from build123d import *

# Parameters (mm, degrees)
F0_R     = 49.4073615008
F1_DEPTH = 21.59
F3_D     = 11.5062
F6_D     = 11.5062


with BuildPart() as f1:
    # F0 (on Front) → F1 (new body)
    with BuildSketch(Plane.XZ):
        Circle(F0_R)
    extrude(amount=F1_DEPTH)

    # F3 (through all)
    with Locations(Plane.XZ.offset(21.59)):
        with Locations((-17.7465770394, 17.1450003982)):
            Hole(F3_D / 2)

    # F6 (through all)
    with Locations(Plane.XZ.offset(21.59)):
        with Locations((15.9418433905, 17.1450003982)):
            Hole(F6_D / 2)


solid = f1.part
Input: part model. Units: mm. Frame: model coordinates. Round coordinates to 2 decimals unless told otherwise and drop trailing zeros. Write each loop counter-clockwise with the first axis right and the second up, starting at its lowest first coordinate (ties: lowest second). Pieces come first, ordered by that corner, then holes.
1) Cut plane A-A (z = 13). Return the cut outline in (x, y), then the cut area to 3 significant figures.
2) Draft query along X for faces 1 (the cylindrical face through (47.126, -10.644, 14.841)), 2 (the cylindrical face through (10.63, -10.64, 14.94)), 3 (the flat face through (-1, -21.59, 1)). Return one class per face: pulls with the +X half, pulls with the -X half, needs draft (parallel to the pull), parting line crosses it, or undercut.
3) Cut plane D-D (z = -14.5). Return the cut outline in (x, y), then the cut area to 3 significant figures.
4) Contact query for flat-ended pins moving along their axis: P1, Ø10.5, axis at x = -17.75, z = 17.15, coming from the +Y side; P2, Ø1, axis at y = -6.5, z = -36.5, coming from the -X side; P3, Ø10, axis at x = 31.5, y = -14.5, coming from the +Z side; P4, Ø12, axis at x = -22.5, y = -17.5, coming from the -Z side. Output: stop coordinate, or through.
5) Cut plane C-C (x = 24.5). Return the cut outline in (y, z).
6) Ray query, L1, parallel to X at y = -13.5, z = 19; L2, parallel to X at y = -18, z = 22; L3, parallel to Z at x = -35, y = -3.75. Return the intervals inside material, ascending.
7) Cut plane B-B (y = -16.75). Return the cut outline in (x, z) (3 decimals), then the cut area to 3 significant figures.
Geometry says:
1. outline: (-47.67, -21.59) - (-21.74, -21.59) - (-21.74, 0) - (-47.67, 0) - close; (-13.76, -21.59) - (11.95, -21.59) - (11.95, 0) - (-13.76, 0) - close; (19.93, -21.59) - (47.67, -21.59) - (47.67, 0) - (19.93, 0) - close
1. area: 1,710 mm2
2. face 1: parting line crosses it
2. face 2: undercut
2. face 3: needs draft
3. outline: (-47.23, -21.59) - (47.23, -21.59) - (47.23, 0) - (-47.23, 0) - close
3. area: 2,040 mm2
4. P1: passes through
4. P2: stops at x = -33.84
4. P3: stops at z = 41.7
4. P4: stops at z = -46.57
5. outline: (-21.59, -42.9) - (0, -42.9) - (0, 42.9) - (-21.59, 42.9) - close
6. L1: x = -45.61 to -23.19, -12.3 to 10.5, 21.39 to 45.61
6. L2: x = -44.24 to -20.83, -14.66 to 12.86, 19.03 to 44.24
6. L3: z = -34.87 to 34.87
7. outline: circle Ø98.815 at (0, 0); hole circle Ø11.506 at (-17.747, 17.145); hole circle Ø11.506 at (15.942, 17.145)
7. area: 7,460 mm2
